Here's how the part is built. I have some questions about the finished solid (model axes, mm). A direction names the side the tool comes from. Round coordinates to 2 decimals unless told otherwise and drop trailing zeros. Write each loop counter-clockwise with the first axis right and the second up, starting at its lowest first coordinate (ties: lowest second). Pieces come first, ordered by that corner, then holes. Notation, with made-up numbers: (25, -38.5) - (61, -38.5) arc R14 ccw to (61, -24.5) - close; hole circle Ø1 at (20, 88). An arc over 180 degrees is marked (long way). Write item = value, one per line. Start each with the question number.
Item 1: Thinking about a two-plate mould opening in X: for faces 1 (the face through (-7.324, 5.944, 44.925)), 2 (the face through (-6.5, 0.2, 37.3)), 3 (the face through (-5, 0, 40)), which applies, pulls with the +X half, pulls with the -X half, needs draft (parallel to the pull), parting line crosses it, or undercut?
Item 2: For P1, Ø4, axis at x = -8, y = 1, coming from the +Z side; P2, Ø4, axis at y = 1.5, z = 45, coming from the +X side; P3, Ø1, axis at y = 7.5, z = 40.5, coming from the +X side; P4, Ø2, axis at y = 3.5, z = 47.5, coming from the +X side (1 decimal), each with a flat end and sliding along its axis, tell me the tip position at first contact or that it passes through.
Item 3: If I drill on line 1 along Y through (x, z) = (1, 44); line 2 along Y through (x, z) = (-6.25, 44.25); line 3 along Z through (x, y) = (-4.25, 3.5), over which ranges is the centre line in solid material (lowest first)? Write a range as [from, to].
Item 4: Which directions (+Z, -Z, +X, -X, +Y, -Y) give clear straight access to the entire face, cutting with the end or side of a thin tool? Please do faces 4 (the face through (-4, 0.5, 39)), 5 (the face through (-5, 10, 40)), 6 (the face through (-9, 2, 44)).
Item 5: If we section it at A-A (y = 3): Please give me the cut outline in (x, z), and give its area (3 significant figures).
```python
from build123d import *

# Parameters (mm, degrees)
SKETCH1_R           = 9.75
BOSS_EXTRUDE5_DEPTH = 2
SKETCH4_R           = 5
BOSS_EXTRUDE6_DEPTH = 8
CUT_EXTRUDE2_DEPTH  = 0.5
FILLET1_R           = 0.5


with BuildPart() as part:
    # Sketch1 → Boss-Extrude5 (new body)
    with BuildSketch(Plane(origin=(0, 0, 0), x_dir=(1, 0, 0), z_dir=(0, 1, 0))):
        with Locations(Location((-5.408676197, -40.3067379, 0), (0, 0, 270))):
            Circle(SKETCH1_R)
    extrude(amount=BOSS_EXTRUDE5_DEPTH)

    # Sketch4 → Boss-Extrude6 (add)
    with BuildSketch(Plane(origin=(0, 2, 0), x_dir=(1, 0, 0), z_dir=(0, 1, 0))):
        with Locations(Location((-5.408676197, -40.3067379, 0), (0, 0, 270))):
            Circle(SKETCH4_R)
    extrude(amount=BOSS_EXTRUDE6_DEPTH)

    # Sketch5 → Cut-Extrude2 (cut)
    with BuildSketch(Plane.XZ):
        with BuildLine():
            Line((-6.676445146, 41.579675489), (-7.817671107, 41.579675489))
            add(Edge.make_bspline(
                [(-7.817671107, 41.579675489), (-7.812310426, 41.695801368), (-7.801825667, 41.922927653), (-7.755267935, 42.253876027), (-7.679847726, 42.565713816), (-7.584651501, 42.861084573), (-7.45766239, 43.136296006), (-7.311142358, 43.396145756), (-7.134259014, 43.635187883), (-6.934371171, 43.853800531), (-6.717385859, 44.05241863), (-6.484125633, 44.223683245), (-6.238533308, 44.369625985), (-5.980560591, 44.488716228), (-5.70970227, 44.580925529), (-5.426730394, 44.648023926), (-5.13074225, 44.688382018), (-4.928974632, 44.692813499), (-4.826685531, 44.695060105)],
                knots=[0, 0, 0, 0, 1.154964179, 2.258951466, 3.315045469, 4.34063582, 5.337653555, 6.322213479, 7.300594401, 8.285733883, 9.262436119, 10.219305053, 11.156568068, 12.097250375, 13.037875795, 13.995471444, 14.983774372, 16, 16, 16, 16], degree=3))
            add(Edge.make_bspline(
                [(-4.826685531, 44.695060105), (-4.719588621, 44.692869366), (-4.50943487, 44.68857053), (-4.203400393, 44.648117964), (-3.913766774, 44.58288823), (-3.640449207, 44.493807864), (-3.383945659, 44.374862374), (-3.14375032, 44.231427232), (-2.922172064, 44.05902337), (-2.717602692, 43.866114214), (-2.536915038, 43.653912553), (-2.373716977, 43.435744039), (-2.238817979, 43.207183965), (-2.125806623, 42.972405889), (-2.038842603, 42.729482892), (-1.977428884, 42.479403561), (-1.940616475, 42.221997964), (-1.935591973, 42.047942984), (-1.933055723, 41.960084143)],
                knots=[0, 0, 0, 0, 1.156722346, 2.269809107, 3.328396062, 4.361258308, 5.3694338, 6.377253737, 7.377324894, 8.397019439, 9.4098266, 10.385180797, 11.337325354, 12.27255833, 13.196816462, 14.119704983, 15.050871513, 16, 16, 16, 16], degree=3))
            add(Edge.make_bspline(
                [(-1.933055723, 41.960084143), (-1.937670931, 41.837184043), (-1.946838122, 41.593067475), (-2.017428332, 41.231911022), (-2.136098747, 40.882386988), (-2.273174428, 40.597782754), (-2.411809943, 40.367733096), (-2.539034806, 40.177847763), (-2.688491104, 39.972524075), (-2.863384002, 39.753136485), (-3.056759049, 39.514665319), (-3.276297862, 39.263262394), (-3.515205381, 38.99383788), (-3.685590507, 38.812419869), (-3.773800915, 38.718497605)],
                knots=[0, 0, 0, 0, 1.155755081, 2.295677249, 3.447123235, 4.6205014, 5.259503175, 5.973005395, 6.77029923, 7.648035671, 8.612336498, 9.658570495, 10.787814065, 12, 12, 12, 12], degree=3))
            Line((-3.773800915, 38.718497605), (-5.987743223, 36.502752412))
            Line((-5.987743223, 36.502752412), (-1.817671107, 36.502752412))
            Line((-1.817671107, 36.502752412), (-1.817671107, 35.464290874))
            Line((-1.817671107, 35.464290874), (-8.163824954, 35.464290874))
            Line((-8.163824954, 35.464290874), (-4.720315338, 39.266574528))
            add(Edge.make_bspline(
                [(-4.720315338, 39.266574528), (-4.638295504, 39.354047762), (-4.480897943, 39.521910498), (-4.259068364, 39.767634589), (-4.058928423, 39.994802676), (-3.879411097, 40.203250768), (-3.725217211, 40.395780628), (-3.592198644, 40.569559806), (-3.48186119, 40.72540892), (-3.367275219, 40.908856301), (-3.253732275, 41.128759827), (-3.157143346, 41.39701125), (-3.099185258, 41.670954142), (-3.090998341, 41.855248913), (-3.086901877, 41.947463951)],
                knots=[0, 0, 0, 0, 1.341560447, 2.574479018, 3.703506985, 4.728875774, 5.651874962, 6.462761537, 7.177175968, 7.787249671, 8.88179658, 9.938774664, 10.968630673, 12, 12, 12, 12], degree=3))
            add(Edge.make_bspline(
                [(-3.086901877, 41.947463951), (-3.087911417, 42.004670669), (-3.089908998, 42.117865747), (-3.117142724, 42.283626365), (-3.155506319, 42.444404941), (-3.214841381, 42.597616639), (-3.286329214, 42.746275734), (-3.375747774, 42.888460482), (-3.483123565, 43.022851966), (-3.602569027, 43.15247391), (-3.734678848, 43.269507844), (-3.874218391, 43.374470164), (-4.022903654, 43.459713223), (-4.176669359, 43.53425977), (-4.340295405, 43.587108395), (-4.509759668, 43.626456912), (-4.686392781, 43.653714425), (-4.806748776, 43.655624226), (-4.868151877, 43.656598566)],
                knots=[0, 0, 0, 0, 0.999432927, 1.977580462, 2.931018689, 3.885672852, 4.844657058, 5.812871023, 6.815890212, 7.849665183, 8.891901864, 9.898878619, 10.897592748, 11.885014695, 12.882178885, 13.896915602, 14.927050508, 16, 16, 16, 16], degree=3))
            add(Edge.make_bspline(
                [(-4.868151877, 43.656598566), (-4.926527495, 43.655401271), (-5.041367662, 43.653045877), (-5.210498233, 43.628743667), (-5.372842642, 43.58917489), (-5.528948546, 43.534289387), (-5.679946595, 43.466576563), (-5.822144632, 43.378854732), (-5.957866841, 43.276807213), (-6.088907502, 43.162274235), (-6.208169616, 43.027904249), (-6.314840719, 42.87528957), (-6.409035513, 42.704263904), (-6.489548923, 42.51512644), (-6.55627432, 42.307380975), (-6.609801194, 42.081280118), (-6.651182642, 41.836725471), (-6.667868533, 41.66694389), (-6.676445146, 41.579675489)],
                knots=[0, 0, 0, 0, 0.911540883, 1.79324023, 2.663162255, 3.518366492, 4.375475705, 5.243419306, 6.122264358, 7.02676621, 7.957780629, 8.921596253, 9.930241338, 11.002848587, 12.128200329, 13.335197372, 14.630280975, 16, 16, 16, 16], degree=3))
        make_face()
    extrude(amount=-CUT_EXTRUDE2_DEPTH, mode=Mode.SUBTRACT)

    # Fillet1
    fillet1_edges = [part.edges().sort_by_distance(p)[0] for p in [
        (-5.408676197, 0, 30.5567379),
        (-5.408676197, 2, 30.5567379),
    ]]
    fillet(fillet1_edges, radius=FILLET1_R)


solid = part.part
```
Reply:
q1.face_1 = parting line crosses it
q1.face_2 = undercut
q1.face_3 = needs draft
q2.P1 = 50.04
q2.P2 = 3.96
q2.P3 = -0.41
q2.P4 = through
q3.line_1 = [0, 2]
q3.line_2 = [0.5, 10]
q3.line_3 = [35.44, 45.17]
q4.face_4 = -Y
q4.face_5 = +Z, -Z, +X, -X, +Y
q4.face_6 = +Y
q5.outline = circle Ø10 at (-5.41, 40.31)
q5.area = 78.5 mm2
